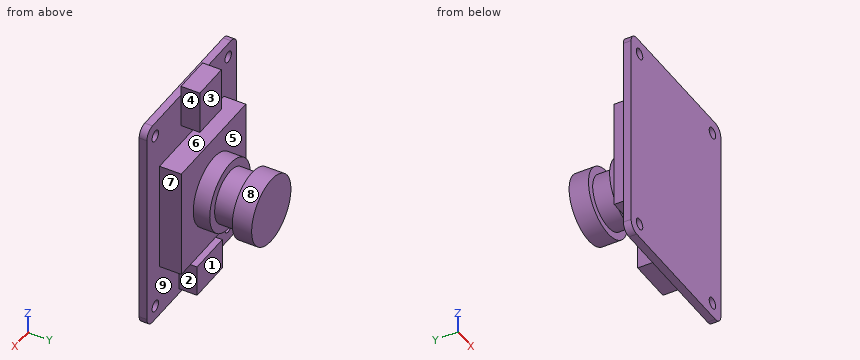
Autodesk Inventor part; units mm, degrees
ref_plane "YZ Plane" through (0, 0, 0) normal (1, 0, 0) x (0, 1, 0)
ref_plane "XZ Plane" through (0, 0, 0) normal (0, 1, 0) x (-1, 0, 0)
ref_plane "XY Plane" through (0, 0, 0) normal (0, 0, 1) x (1, 0, 0)
sketch "スケッチ1" plane through (0, 0, 0) normal (0, 1, 0) x (-1, 0, 0)
  line L0 (0, 0) -> (32, 0)
  line L1 (32, 0) -> (32, -45)
  line L2 (32, -45) -> (0, -45)
  line L3 (0, -45) -> (0, 0)
  circle A0 centre (29, -3) radius 1.15
  circle A1 centre (29, -42) radius 1.15
  circle A2 centre (3, -3) radius 1.15
  circle A3 centre (3, -42) radius 1.15
  dimension "d0" = 45
  dimension "d1" = 32
  dimension "d2" = 2.3
  dimension "d3" = 2.3
  dimension "d4" = 2.3
  dimension "d5" = 2.3
  dimension "d16" = 39
  dimension "d17" = 26
  dimension "d18" = 3
  dimension "d19" = 3
  dimension "d20" = 26
  dimension "d21" = 39
extrude "押し出し1" add sketch "スケッチ1" along normal blind 1.6
sketch "スケッチ2" plane through (0, 1.6, 0) normal (0, 1, 0) x (1, 0, 0)
  line L0 (-20.5, 37.5) -> (-11.5, 37.5)
  line L1 (-11.5, 37.5) -> (-11.5, 44)
  line L2 (-11.5, 44) -> (-20.5, 44)
  line L3 (-20.5, 44) -> (-20.5, 37.5)
  line L4 (-19.85, -2) -> (-12.15, -2)
  line L5 (-12.15, -2) -> (-12.15, 7)
  line L6 (-12.15, 7) -> (-19.85, 7)
  line L7 (-19.85, 7) -> (-19.85, -2)
  line L8 (-27.5, 11) -> (-4.5, 11)
  line L9 (-4.5, 11) -> (-4.5, 34)
  line L10 (-4.5, 34) -> (-27.5, 34)
  line L11 (-27.5, 34) -> (-27.5, 11)
  line L12 (0, 45) -> (-32, 45)
  line L13 (-32, 0) -> (0, 0)
  line L14 (-16, 0) -> (-16, 45) construction
  line L15 (-1.3785, 22.5) -> (-33.3785, 22.5) construction
  line L16 (-32, 45) -> (-32, 0)
  dimension "d22" = 9
  dimension "d23" = 7.7
  dimension "d25" = 23
  dimension "d26" = 23
  dimension "d27" = 9
  dimension "d28" = 6.5
  dimension "d29" = 1
  dimension "d30" = 2
  dimension "d31" = 11.5
  dimension "d32" = 11.5
  dimension "d33" = 3.85
  dimension "d34" = 4.5
  dimension "d35" = 22.5
  dimension "d36" = 45
fillet "フィレット1" radius 2 4 edges at (-32, 0.8, -45) (0, 0.8, -45) (-32, 0.8, 0) (0, 0.8, 0)
extrude "押し出し2" add sketch "スケッチ2" along normal blind 3.9 contours L7 L13 L5 L4 | L7 L6 L5 L13
sketch "スケッチ3" plane through (0, 1.6, 0) normal (0, 1, 0) x (1, 0, 0)
  line L0 (-20.5, 37.5) -> (-11.5, 37.5)
  line L1 (-11.5, 37.5) -> (-11.5, 44)
  line L2 (-11.5, 44) -> (-20.5, 44)
  line L3 (-20.5, 44) -> (-20.5, 37.5)
  line L4 (-19.85, -2) -> (-12.15, -2)
  line L5 (-12.15, -2) -> (-12.15, 7)
  line L6 (-12.15, 7) -> (-19.85, 7)
  line L7 (-19.85, 7) -> (-19.85, -2)
  line L8 (-27.5, 11) -> (-4.5, 11)
  line L9 (-4.5, 11) -> (-4.5, 34)
  line L10 (-4.5, 34) -> (-27.5, 34)
  line L11 (-27.5, 34) -> (-27.5, 11)
  line L12 (0, 45) -> (-32, 45)
  line L13 (-32, 0) -> (0, 0)
  line L14 (-16, 0) -> (-16, 45) construction
  line L15 (-1.3785, 22.5) -> (-33.3785, 22.5) construction
  line L16 (-32, 45) -> (-32, 0)
  dimension "d39" = 9
  dimension "d40" = 7.7
  dimension "d41" = 23
  dimension "d42" = 23
  dimension "d43" = 9
  dimension "d44" = 6.5
  dimension "d45" = 1
  dimension "d46" = 2
  dimension "d47" = 11.5
  dimension "d48" = 11.5
  dimension "d49" = 3.85
  dimension "d50" = 4.5
  dimension "d51" = 22.5
  dimension "d52" = 45
extrude "押し出し3" add sketch "スケッチ3" along normal blind 3.7 contours L3 L2 L1 L0
sketch "スケッチ4" plane through (0, 1.6, 0) normal (0, 1, 0) x (1, 0, 0)
  line L0 (-20.5, 37.5) -> (-11.5, 37.5)
  line L1 (-11.5, 37.5) -> (-11.5, 44)
  line L2 (-11.5, 44) -> (-20.5, 44)
  line L3 (-20.5, 44) -> (-20.5, 37.5)
  line L4 (-19.85, -2) -> (-12.15, -2)
  line L5 (-12.15, -2) -> (-12.15, 7)
  line L6 (-12.15, 7) -> (-19.85, 7)
  line L7 (-19.85, 7) -> (-19.85, -2)
  line L8 (-27.5, 11) -> (-4.5, 11)
  line L9 (-4.5, 11) -> (-4.5, 34)
  line L10 (-4.5, 34) -> (-27.5, 34)
  line L11 (-27.5, 34) -> (-27.5, 11)
  line L12 (0, 45) -> (-32, 45)
  line L13 (-32, 0) -> (0, 0)
  line L14 (-16, 0) -> (-16, 45) construction
  line L15 (-1.3785, 22.5) -> (-33.3785, 22.5) construction
  line L16 (-32, 45) -> (-32, 0)
  dimension "d55" = 9
  dimension "d56" = 7.7
  dimension "d57" = 23
  dimension "d58" = 23
  dimension "d59" = 9
  dimension "d60" = 6.5
  dimension "d61" = 1
  dimension "d62" = 2
  dimension "d63" = 11.5
  dimension "d64" = 11.5
  dimension "d65" = 3.85
  dimension "d66" = 4.5
  dimension "d67" = 22.5
  dimension "d68" = 45
extrude "押し出し4" add sketch "スケッチ4" along normal blind 4.5 contours L11 L10 L9 L8
sketch "スケッチ5" plane through (0, 6.1, 0) normal (0, 1, 0) x (1, 0, 0)
  circle A0 centre (-16, 22.5) radius 7.25
  line L0 (0, 2) -> (0, 43)
  point P0 (0, 0)
  dimension "d71" = 14.5
  dimension "d72" = 22.5
  dimension "d73" = 16
extrude "押し出し5" add sketch "スケッチ5" along normal blind 3.4
sketch "スケッチ6" plane through (-16, 9.5, -22.5) normal (0, 1, 0) x (1, 0, 0)
  circle A0 centre (0, 0) radius 5.5
  circle A1 centre (0, 0) radius 7.25
  point P0 (16, -22.5)
  dimension "d76" = 11
extrude "押し出し6" add sketch "スケッチ6" along normal blind 4.5 contours A0
sketch "スケッチ7" plane through (-16, 14, -22.5) normal (0, 1, 0) x (1, 0, 0)
  circle A0 centre (0, 0) radius 7
  circle A1 centre (0, 0) radius 5.5
  point P0 (16, -22.5)
  dimension "d79" = 14
extrude "押し出し7" add sketch "スケッチ7" along normal blind 4 contours A0 | A1
equation "\"d3\" = d2"
equation "\"d4\" = d2"
equation "\"d5\" = d2"
equation "\"d20\" = d17"
equation "\"d21\" = d16"
equation "\"d31\" = 0.5 * d25"
equation "\"d32\" = 0.5 * d26"
equation "\"d33\" = 0.5 * d23"
equation "\"d34\" = 0.5 * d22"
equation "\"d35\" = 0.5 * d36"
equation "\"d47\" = 0.5 * d41"
equation "\"d48\" = 0.5 * d42"
equation "\"d49\" = 0.5 * d40"
equation "\"d50\" = 0.5 * d39"
equation "\"d51\" = 0.5 * d52"
equation "\"d63\" = 0.5 * d57"
equation "\"d64\" = 0.5 * d58"
equation "\"d65\" = 0.5 * d56"
equation "\"d66\" = 0.5 * d55"
equation "\"d67\" = 0.5 * d68"
properties part number "KCSU5380"
The listing builds one solid part. Answer for the finished solid, in the listing's coordinates (mm). Face numbers are marked on the shaded views. A direction names the side the tool comes from. Give positions to 0.01 mm unless a question says otherwise; leave off trailing zeros. Write each loop counter-clockwise with the first axis right and the second up, starting at its lowest first coordinate (ties: lowest second). Pieces come first, ordered by that corner, then holes.
1) Section A-A (z = -3) is taken. Write down the section's boundary in (x, y).
2) A tool of negligible diameter and unlimited length cuts with its end or side. For the marked faces 1, 2, 3, 4 and 5, from which of +Z, -Z, +X, -X, +Y, -Y can it reach the whole face along a straight path? Write none if from no direction.
3) For a pull along Z with two mould halves and no side action, classify the marked faces 6, 7, 8 and 9 as pulls with the +Z half, pulls with the -Z half, needs draft (parallel to the pull), parting line crosses it, or undercut.
4) Find the intervals of material crossed by L1, parallel to Z at x = -29, y = 0.55; L2, parallel to Z at x = -14, y = 3.75; L3, parallel to Y at x = -27.5, z = -36.5, in increasing order.
5) Section D-D (x = -16) is taken. Write down the section's boundary in (y, z).
6) Given P1, Ø1.2, axis at y = 3, z = -4.5, coming from the +X side; P2, Ø5, axis at y = 3, z = -20, coming from the +X side; P3, Ø4, axis at x = -24, z = -34.5, coming from the +Y side; P4, Ø0.6, axis at x = -14.5, z = 1.5, coming from the -Y side, each flat-ended and moving along its own axis, determine where each tip first touches the part or whether it passes through.
7) Section B-B (x = -3) is taken. Write down the section's boundary in (y, z), and give its area (3 significant figures).
8) Section C-C (y = 3) is taken. Write down the section's boundary in (x, z).
Response:
1. outline: (-32, 0) - (-30.15, 0) - (-30.15, 1.6) - (-32, 1.6) - close; (-27.85, 0) - (-4.15, 0) - (-4.15, 1.6) - (-12.15, 1.6) - (-12.15, 5.5) - (-19.85, 5.5) - (-19.85, 1.6) - (-27.85, 1.6) - close; (-1.85, 0) - (0, 0) - (0, 1.6) - (-1.85, 1.6) - close
2. face 1: -Z, +X, -X, +Y
2. face 2: -Z, +X, +Y
2. face 3: +Z, +X, -X, +Y
2. face 4: +Z, +X, +Y
2. face 5: +Y
3. face 6: undercut
3. face 7: needs draft
3. face 8: parting line crosses it
3. face 9: undercut
4. L1: z = -45 to -43.15, -40.85 to -4.15, -1.85 to 0
4. L2: z = -44 to -37.5, -34 to -11, -7 to 2
4. L3: y = 0 to 1.6
5. outline: (0, -45) - (1.6, -45) - (1.6, -44) - (5.3, -44) - (5.3, -37.5) - (1.6, -37.5) - (1.6, -34) - (6.1, -34) - (6.1, -29.75) - (9.5, -29.75) - (9.5, -28) - (14, -28) - (14, -29.5) - (18, -29.5) - (18, -15.5) - (14, -15.5) - (14, -17) - (9.5, -17) - (9.5, -15.25) - (6.1, -15.25) - (6.1, -11) - (1.6, -11) - (1.6, -7) - (5.5, -7) - (5.5, 2) - (1.6, 2) - (1.6, 0) - (0, 0) - close
6. P1: stops at x = -12.15
6. P2: stops at x = 0
6. P3: stops at y = 6.1
6. P4: stops at y = 1.6
7. outline: (0, -45) - (1.6, -45) - (1.6, -43.15) - (0, -43.15) - close; (0, -40.85) - (1.6, -40.85) - (1.6, -4.15) - (0, -4.15) - close; (0, -1.85) - (1.6, -1.85) - (1.6, 0) - (0, 0) - close
7. area: 64.6 mm2
8. outline: (-27.5, -34) - (-4.5, -34) - (-4.5, -11) - (-27.5, -11) - close; (-20.5, -44) - (-11.5, -44) - (-11.5, -37.5) - (-20.5, -37.5) - close; (-19.85, -7) - (-12.15, -7) - (-12.15, 2) - (-19.85, 2) - close
